Autodesk Fusion 360 part; units mm, degrees
sketch "Sketch1" plane through (0, 0, 0) normal (0, 0, 1) x (1, 0, 0)
  line L0 (-54.7772, 22.5) -> (-54.7772, -22.5)
  line L1 (-54.7772, -22.5) -> (-67.7772, -22.5)
  ellipse E0 centre (0, 0) end of major axis (-70, 0) minor radius 90
  line L2 (70, 0) -> (-70, 0) construction
  line L3 (-54.7772, 22.5) -> (-67.7772, 22.5)
  line L4 (0, 0) -> (70, 0) construction
  line L5 (0, 0) -> (0, 90) construction
  line L6 (54.7772, 22.5) -> (54.7772, -22.5)
  line L7 (54.7772, -22.5) -> (67.7772, -22.5)
  line L8 (54.7772, 22.5) -> (67.7772, 22.5)
  dimension "d2" = 45
  dimension "d29" = 13
  dimension "d30" = 70
  dimension "d31" = 90
  dimension "d32" = 13
extrude "Extrude1" add sketch "Sketch1" along normal blind 3 contours L0 L1 E0 L3 L6 L7 L8
sketch "Sketch2" plane through (0, 0, 3) normal (0, 0, 1) x (-1, 0, 0)
  line L0 (54.7772, -22.5) -> (54.7772, 22.5)
  line L1 (67.7772, -22.5) -> (54.7772, -22.5)
  ellipse E0 centre (0, 0) end of major axis (0, 90) minor radius 70 (-67.7772, -22.5) -> (67.7772, -22.5) ccw
  line L2 (54.7772, 22.5) -> (67.7772, 22.5)
  line L3 (-54.7772, 22.5) -> (-54.7772, -22.5)
  line L4 (-54.7772, -22.5) -> (-67.7772, -22.5)
  ellipse E1 centre (0, 0) end of major axis (0, 90) minor radius 70 (67.7772, 22.5) -> (-67.7772, 22.5) ccw
  line L5 (-67.7772, 22.5) -> (-54.7772, 22.5)
  ellipse E2 centre (0, 0) end of major axis (68.5, 0) minor radius 86.5
  line L6 (-68.5, 0) -> (68.5, 0) construction
  line L7 (0, -86.5) -> (0, 86.5) construction
  ellipse E3 centre (0, 0) end of major axis (66, 0) minor radius 85
  line L8 (-66, 0) -> (66, 0) construction
  line L9 (0, -85) -> (0, 85) construction
  dimension "d33" = 137
  dimension "d34" = 173
  dimension "d35" = 132
  dimension "d36" = 170
extrude "Extrude2" cut sketch "Sketch2" against normal blind 1.5 contours L1 L2 E2 E3 | L1 L4 E2 E3 | L2 L5 E2 E3 | L4 L5 E2 E3
sketch "Sketch3" plane through (0, 0, 3) normal (0, 0, 1) x (-1, 0, 0)
  line L0 (21, -76) -> (-21, -76)
  line L1 (-21, -76) -> (-21, -34)
  line L2 (-21, -34) -> (21, -34)
  line L3 (21, -34) -> (21, -76)
  line L4 (63.6457, -22.5) -> (54.7772, -22.5)
  line L5 (54.7772, 22.5) -> (63.6457, 22.5)
  line L6 (54.7772, -22.5) -> (54.7772, 22.5)
  line L7 (-54.7772, 22.5) -> (-54.7772, -22.5)
  line L8 (-54.7772, -22.5) -> (-63.6457, -22.5)
  line L9 (-63.6457, 22.5) -> (-54.7772, 22.5)
  ellipse E0 centre (0, 0) end of major axis (0, 85) minor radius 66 (63.6457, 22.5) -> (-63.6457, 22.5) ccw
  ellipse E1 centre (0, 0) end of major axis (0, 85) minor radius 66 (-63.6457, -22.5) -> (63.6457, -22.5) ccw
  line L10 (-34.7974, -11.3414) -> (-54.7974, -11.3414)
  line L11 (-54.7974, -11.3414) -> (-54.7974, 48.6586)
  line L12 (-54.7974, 48.6586) -> (-34.7974, 48.6586)
  line L13 (-34.7974, 48.6586) -> (-34.7974, -11.3414)
  line L14 (54.9535, -10.6734) -> (34.9535, -10.6734)
  line L15 (34.9535, -10.6734) -> (34.9535, 49.3266)
  line L16 (34.9535, 49.3266) -> (54.9535, 49.3266)
  line L17 (54.9535, 49.3266) -> (54.9535, -10.6734)
  line L18 (-20.5, 0) -> (20.5, 0)
  line L19 (20.5, 0) -> (20.5, 76)
  line L20 (20.5, 76) -> (-20.5, 76)
  line L21 (-20.5, 76) -> (-20.5, 0)
  line L22 (38.1039, 52.22) -> (23.1039, 52.22)
  line L23 (23.1039, 52.22) -> (23.1039, 62.22)
  line L24 (23.1039, 62.22) -> (38.1039, 62.22)
  line L25 (38.1039, 62.22) -> (38.1039, 52.22)
  circle A0 centre (162.6967, 56.966) radius 52
  line L26 (0, 0) -> (0, 100)
  dimension "d21" = 42
  dimension "d22" = 42
  dimension "d37" = 20
  dimension "d38" = 60
  dimension "d39" = 20
  dimension "d40" = 60
  dimension "d41" = 41
  dimension "d42" = 76
  dimension "d43" = 15
  dimension "d44" = 10
  dimension "d45" = 104
  dimension "d46" = 100
  dimension "d47" = 20.5
  dimension "d48" = 21
  dimension "d49" = 34
extrude "Extrude3" cut sketch "Sketch3" against normal blind 0.5 contours L0 L1 L2 L3 | L18 L19 L20 L26 | L18 L20 L21 L26 | L5 L6 E0 L14 L15 L16 L17 | L7 L9 E0 L10 L11 L12 L13
extrude "Extrude4" cut sketch "Sketch3" against normal blind 3 contours L22 L23 L24 L25
The model under review builds one solid part; all positions refer to its coordinate system, in mm. A direction names the side the tool comes from. Give positions to 0.01 mm unless a question says otherwise; leave off trailing zeros. Loops run counter-clockwise (first coordinate to the right, second up) from the corner with the lowest first, then second, coordinate; pieces in that order, holes last. Notation, with made-up numbers: (53, 82.5) -> (59, 82.5) arc R22 ccw to (59, 93.5) -> close; hole circle Ø5 at (41, -1). An arc over 180 degrees is marked (long way). Put each result on its own line as item: value. Start each with the question number.
1. We need section A-A on y = -15. State the section outline as (x, z) points.
2. Clearance check with flat-ended pins moving along their axes: P1, Ø1.5, axis at y = 4, z = 2, coming from the -X side; P2, Ø0.6, axis at x = -47.5, z = 3, coming from the +Y side; P3, Ø22, axis at x = 48.5, y = -10, coming from the +Z side. State where each tip first meets the part, or that it passes through.
3. Wall thickness on probe 1 along X at (y, z) = (62.5, 2.05); probe 2 along X at (y, z) = (-30.5, 2.1); probe 3 along X at (y, z) = (67, 2.55): over which ranges is each line inside the solid? List them lowest first.
4. Mouldability with a two-part tool opening along Y and no side actions: class faces 3 (the face through (0.3, 85.2, 1.5)), 4 (the face through (-1, 1, 0)), 5 (the face through (-45, -20, 2.5)) as released by +Y, released by -Y, zero draft, split by the parting line, or undercut.
5. For faces 1 (the face through (0, 55, 2.5)), 2 (the face through (-1, 20, 3)), list the 3-axis set-ups (+Z, -Z, +X, -X, +Y, -Y) from which the entire face can be reached by the end or side of a thin tool; tool diameter is ignored.
Determined:
1. outline: (-54.78, 0) -> (54.78, 0) -> (54.78, 2.5) -> (34.8, 2.5) -> (34.8, 3) -> (20.5, 3) -> (20.5, 2.5) -> (-20.5, 2.5) -> (-20.5, 3) -> (-34.95, 3) -> (-34.95, 2.5) -> (-54.78, 2.5) -> close
2. P1: x = -54.78
2. P2: y = 66.46
2. P3: z = 2.5
3. probe 1: -50.37 to -47.36, -44.73 to 44.73, 47.36 to 50.37
3. probe 2: -65.86 to -64.1, -61.6 to 61.6, 64.1 to 65.86
3. probe 3: -46.74 to -43.33, -40.61 to -21, 21 to 40.61, 43.33 to 46.74
4. face 3: undercut
4. face 4: zero draft
4. face 5: undercut
5. face 1: +Z
5. face 2: +Z, +X, -X, +Y, -Y
